The model under review builds one solid part; all positions refer to its coordinate system, in mm. A direction names the side the tool comes from. Round coordinates to 2 decimals unless told otherwise and drop trailing zeros. Write each loop counter-clockwise with the first axis right and the second up, starting at its lowest first coordinate (ties: lowest second). Pieces come first, ordered by that corner, then holes. Notation, with made-up numbers: (-3, 80.5) -> (56, 80.5) arc R23 ccw to (56, 91.5) -> close; hole circle Ø6 at (33, -34.75). An arc over 180 degrees is marked (long way). Answer as a JSON object with one key per item and string values. Group by question number.
1) To check wall thickness, follow probe 1 along Y at (x, z) = (0, 0.85); probe 2 along Y at (x, z) = (-3, 0.55); probe 3 along Z at (x, y) = (11, 11). State the ranges of each line that lie inside material, in increasing order. Write a range as [from, to].
2) Mouldability with a two-part tool opening along X and no side actions: class faces 5 (the flat face through (3.24, 0, 3)), 6 (the flat face through (14, 33, 1)), 7 (the cylindrical face through (29.7, 31.06, 0.69)) as pulls with the +X half, pulls with the -X half, needs draft (parallel to the pull), parting line crosses it, or undercut.
3) Insertion check: pin 1 Ø1.8 at (x, y) = (28, 28) entering from -Z; pin 2 Ø3 at (x, z) = (8.5, 4) entering from +Y; pin 3 Ø3 at (y, z) = (0.5, 4) entering from -X. Each pin has a flat end and moves straight along its axis. Give the tip position at first contact, or say it passes through.
4) We need section C-C, the plane y = 14. Write out the cut boundary in (x, z).
5) Machinability: for faces 1 (the flat face through (7, 2.28, 3)), 2 (the cylindrical face through (8.445, 18.259, -7.888)), 3 (the flat face through (7, -1.53, 3)), 4 (the flat face through (10.8, 0, 3)), which of the approach directions +Z, -Z, +X, -X, +Y, -Y give a long, thin tool a straight path to every point of the face, cutting with its end or side? Answer none if there is none.
6) We need section B-B, the plane x = 4. Write out the cut boundary in (y, z).
7) We need section A-A, the plane y = 28. Write out the cut boundary in (x, z), then the cut area to 3 significant figures.
from build123d import *

# Parameters (mm, degrees)
SKETCH1_W           = 38
SKETCH1_H           = 38
SKETCH1_R           = 1.3
SKETCH1_R_2         = 0.7
BOSS_EXTRUDE1_DEPTH = 1.4
SKETCH2_W           = 7.56
SKETCH2_H           = 3.81
BOSS_EXTRUDE2_DEPTH = 4
SKETCH3_R           = 7
BOSS_EXTRUDE3_DEPTH = 16


with BuildPart() as part:
    # Sketch1 → Boss-Extrude1 (new body)
    # profile 1 of 2: a face of its own
    with BuildSketch(Plane.XY):
        with Locations((14, 14)):
            Rectangle(SKETCH1_W, SKETCH1_H)
        with Locations((-3, -3)):
            Circle(SKETCH1_R, mode=Mode.SUBTRACT)
        with Locations((31, -3)):
            Circle(SKETCH1_R, mode=Mode.SUBTRACT)
        with Locations((31, 31)):
            Circle(SKETCH1_R, mode=Mode.SUBTRACT)
        with Locations((-3, 31)):
            Circle(SKETCH1_R, mode=Mode.SUBTRACT)
        with BuildLine():
            ThreePointArc((0.1, 29.3), (-0.889949494, 28.889949494), (-1.3, 27.9))
            Line((-1.3, 27.9), (-1.3, 0.1))
            ThreePointArc((-1.3, 0.1), (-0.889949494, -0.889949494), (0.1, -1.3))
            Line((0.1, -1.3), (27.9, -1.3))
            ThreePointArc((27.9, -1.3), (28.889949494, -0.889949494), (29.3, 0.1))
            Line((29.3, 0.1), (29.3, 27.9))
            ThreePointArc((29.3, 27.9), (28.889949494, 28.889949494), (27.9, 29.3))
            Line((27.9, 29.3), (0.1, 29.3))
        make_face(mode=Mode.SUBTRACT)
    # profile 2 of 2: a face of its own
    with BuildSketch(Plane.XY):
        with BuildLine():
            Line((0.1, 29.3), (27.9, 29.3))
            ThreePointArc((27.9, 29.3), (28.889949494, 28.889949494), (29.3, 27.9))
            Line((29.3, 27.9), (29.3, 0.1))
            ThreePointArc((29.3, 0.1), (28.889949494, -0.889949494), (27.9, -1.3))
            Line((27.9, -1.3), (0.1, -1.3))
            ThreePointArc((0.1, -1.3), (-0.889949494, -0.889949494), (-1.3, 0.1))
            Line((-1.3, 0.1), (-1.3, 27.9))
            ThreePointArc((-1.3, 27.9), (-0.889949494, 28.889949494), (0.1, 29.3))
        make_face()
        with Locations((0, 28)):
            Circle(SKETCH1_R_2, mode=Mode.SUBTRACT)
        with Locations((28, 28)):
            Circle(SKETCH1_R_2, mode=Mode.SUBTRACT)
        Circle(SKETCH1_R_2, mode=Mode.SUBTRACT)
        with Locations((28, 0)):
            Circle(SKETCH1_R_2, mode=Mode.SUBTRACT)
    extrude(amount=BOSS_EXTRUDE1_DEPTH)

    # Sketch2 → Boss-Extrude2 (add)
    with BuildSketch(Plane.XY.offset(1.4)):
        with Locations((7.02, 0.375)):
            Rectangle(SKETCH2_W, SKETCH2_H)
    extrude(amount=BOSS_EXTRUDE2_DEPTH)

    # Sketch3 → Boss-Extrude3 (add)
    with BuildSketch(Plane(origin=(0, 0, 0), x_dir=(-1, 0, 0), z_dir=(0, 0, -1))):
        with Locations(Location((-14, 14, 0), (0, 0, 180))):
            Circle(SKETCH3_R)
    extrude(amount=BOSS_EXTRUDE3_DEPTH)


solid = part.part
Here are the results:
{
 "1": {"probe 1": "y = [-5, -0.7], [0.7, 27.3], [28.7, 33]", "probe 2": "y = [-5, -4.3], [-1.7, 29.7], [32.3, 33]", "probe 3": "z = [-16, 1.4]"},
 "2": {"face 5": "pulls with the -X half", "face 6": "needs draft", "face 7": "undercut"},
 "3": {"pin 1": "stops at z = 0", "pin 2": "stops at y = 2.28", "pin 3": "stops at x = 3.24"},
 "4": {"outline": "(-5, 0) -> (7, 0) -> (7, -16) -> (21, -16) -> (21, 0) -> (33, 0) -> (33, 1.4) -> (-5, 1.4) -> close"},
 "5": {"face 1": "+Z, +X, -X, +Y", "face 2": "-Z", "face 3": "+Z, +X, -X, -Y", "face 4": "+Z, +X, +Y, -Y"},
 "6": {"outline": "(-5, 0) -> (33, 0) -> (33, 1.4) -> (2.28, 1.4) -> (2.28, 5.4) -> (-1.53, 5.4) -> (-1.53, 1.4) -> (-5, 1.4) -> close"},
 "7": {"outline": "(-5, 0) -> (-0.7, 0) -> (-0.7, 1.4) -> (-5, 1.4) -> close; (0.7, 0) -> (27.3, 0) -> (27.3, 1.4) -> (0.7, 1.4) -> close; (28.7, 0) -> (33, 0) -> (33, 1.4) -> (28.7, 1.4) -> close", "area": "49.3 mm^2"}
}
